Could you check a few things on this drawing? It's one solid part, dimensions in mm from its lowest x, y, z. A direction names the side the tool comes from. Coordinates: 2 decimals unless noted, no trailing zeros. Loops run counter-clockwise (first coordinate to the right, second up) from the corner with the lowest first, then second, coordinate; pieces in that order, holes last. Notation, with made-up numbers: M 39,-27.5 L 53,-27.5 A17 cw 53,-17.5 Z; hole C -28.75,-33.75 d5. An arc over 180 degrees is marked long. Use one line per item in the form item = value. Start each with the question number.
(1) Imagine slicing it at B-B, the plane y = 19.5. Please give me the cut outline in (x, z) (3 decimals).
(2) Will these pins go through, and if not, where does the flat tip stop? P1, Ø8, axis at x = 8, y = 2.5, coming from the +Z side (3 decimals); P2, Ø2, axis at y = 9, z = 161.5, coming from the +X side (3 decimals); P3, Ø10, axis at x = 16.5, y = 5.5, coming from the +Z side; P4, Ø6, axis at y = 3.5, z = 83.5, coming from the -X side.
(3) Please list where these lines run through material, in increasing order: L1, parallel to Y at x = 11.25, z = 68.5 (3 decimals); L2, parallel to Z at x = 19.25, y = 24 (3 decimals).
(4) On a 3-axis mill with a long thin cutter (end or side, diameter ignored), from which of +Z, -Z, +X, -X, +Y, -Y can I reach the whole of each face in a straight line? I mean the marked faces 4 and 5. Say none if no direction works.
(5) Imagine slicing it at A-A, the plane z = 29. Please give me the cut outline in (x, y) (3 decimals), and give its area (3 significant figures).
(6) Imagine slicing it at C-C, the plane x = 11.25. Please give me the cut outline in (y, z) (3 decimals), and give its area (3 significant figures).
(7) Thinking about a two-plate mould opening in X: for the marked faces 1, 2 and 3, which applies, +X half, -X half, draft (parallel to the pull), parting line (faces both ways), or undercut?
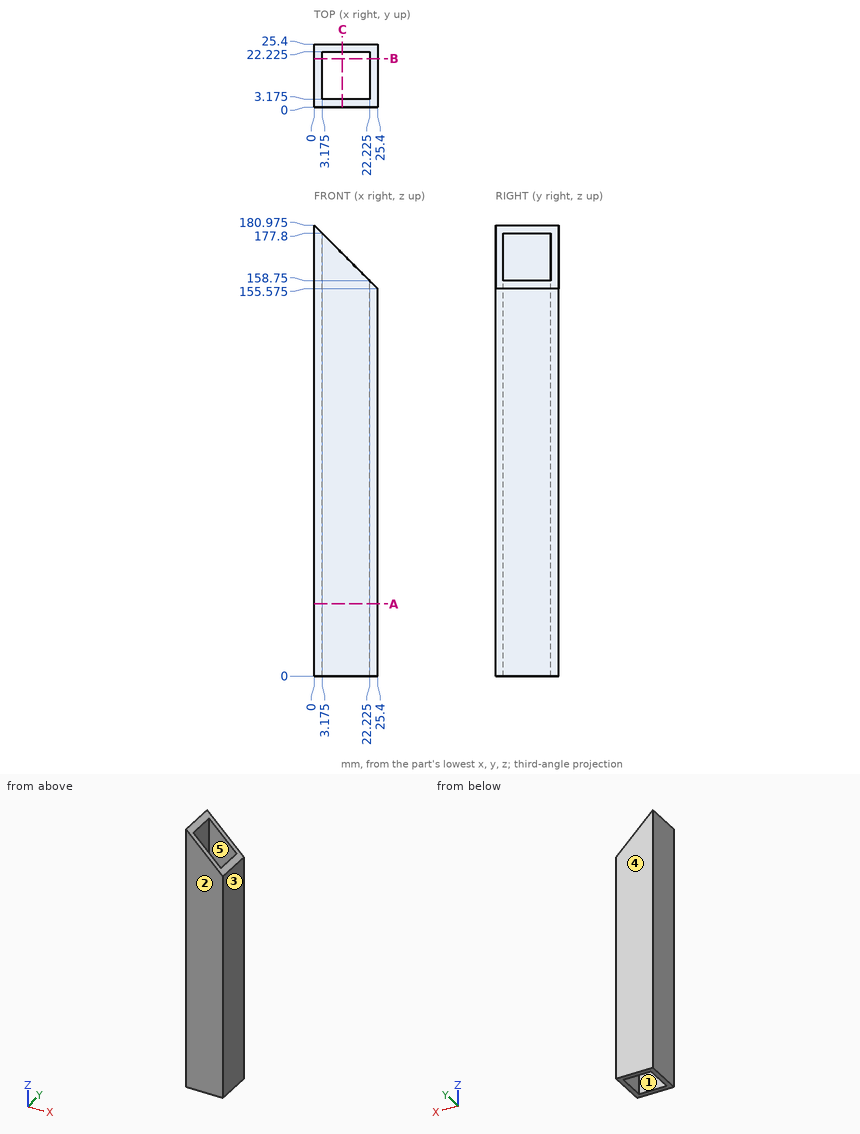
Answer:
q1.outline = M 0,0 L 3.175,0 L 3.175,177.8 L 0,180.975 Z; M 22.225,0 L 25.4,0 L 25.4,155.575 L 22.225,158.75 Z
q2.P1 = 176.975
q2.P2 = 3.175
q2.P3 = 168.9
q2.P4 = 0
q3.L1 = 0 to 3.175, 22.225 to 25.4
q3.L2 = 0 to 161.725
q4.face_4 = +Z, -Z, +X, -X, +Y
q4.face_5 = +Z, -Z
q5.outline = M 0,0 L 25.4,0 L 25.4,25.4 L 0,25.4 Z; hole M 3.175,3.175 L 22.225,3.175 L 22.225,22.225 L 3.175,22.225 Z
q5.area = 282 mm²
q6.outline = M 0,0 L 3.175,0 L 3.175,169.725 L 0,169.725 Z; M 22.225,0 L 25.4,0 L 25.4,169.725 L 22.225,169.725 Z
q6.area = 1,080 mm²
q7.face_1 = undercut
q7.face_2 = draft
q7.face_3 = +X half
